Autodesk Inventor part; units mm, degrees
ref_plane "YZ Plane" through (0, 0, 0) normal (1, 0, 0) x (0, 1, 0)
ref_plane "XY Plane" through (0, 0, 0) normal (0, 0, 1) x (1, 0, 0)
sketch "Sketch1" plane through (0, 0, 0) normal (1, 0, 0) x (0, 1, 0)
  line L0 (0, -54.8873) -> (0, 55.2482)
  line L1 (0, 55.8624) -> (24.75, 55.8624)
  line L2 (24.75, 55.8624) -> (24.75, -93.6376)
  line L3 (24.75, -93.6376) -> (7.5, -93.6376)
  line L4 (7.5, -93.6376) -> (7.5, -96.6376)
  line L5 (7.5, -96.6376) -> (10, -98.6376)
  line L6 (10, -98.6376) -> (10, -99.6376)
  line L7 (10, -99.6376) -> (0, -99.6376)
  line L8 (0, -99.6376) -> (0, 55.8624)
  point P0 (0, 0)
  dimension "d0" = 155.5
  dimension "d1" = 24.75
  dimension "d2" = 7.5
  dimension "d3" = 10
  dimension "d4" = 6
  dimension "d5" = 1
  dimension "d6" = 2
revolve "Revolution1" add sketch "Sketch1" angle 360 about axis through (0, 0, -54.8873) along (0, 0, 1)
hole "Hole1" at (0, 0, -99.6376) direction (0, 0, 1) diameter 6 depth 53.5
properties part number "solenoid_body"
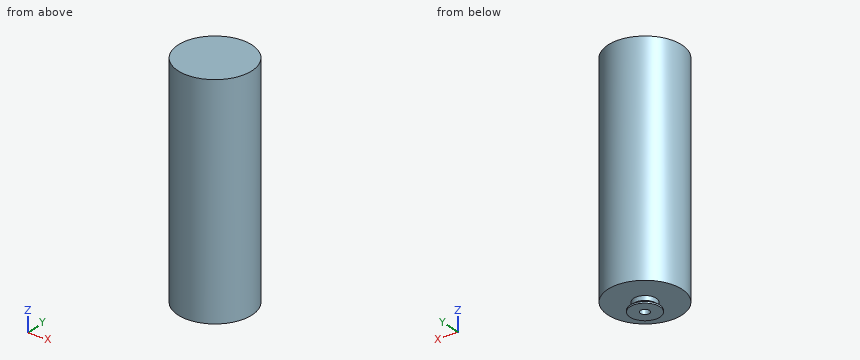
Design review of the part built by this model. Coordinates are the model's own, in mm. Give positions to 0.01 mm unless a question says otherwise; leave off trailing zeros. Order: outer loops, then holes, each group sorted by start corner. A loop starts at its lowest first (then second) coordinate and runs counter-clockwise, first axis right, second up. Notation, with made-up numbers: (8.5, 4.25) - (25.5, 4.25) arc R35 cw to (25.5, 42.25) - close; hole circle Ø1 at (34.5, 33). An arc over 180 degrees is marked (long way). Use a Markdown table: item, result. Add a question column.
(1) Clearance check with flat-ended pins moving along their axes: P1, Ø6, axis at y = 1.5, z = 0, coming from the -X side; P2, Ø1, axis at x = 14.5, z = -44, coming from the -Y side; P3, Ø3, axis at y = 12.5, z = -81, coming from the +X side; P4, Ø15, axis at x = 11, y = 5.5, coming from the -Z side. State where each tip first meets the part, or that it passes through.
(2) Wall thickness on probe 1 along X at (y, z) = (0, -71); probe 2 along Z at (x, y) = (12, -16.5): over which ranges is each line inside the solid? List them lowest first. Write a range as [from, to].
(3) Add section D-D on z = -12.5. Give the boundary of the cut face in (x, y).
(4) Add section A-A on y = 0. Give the boundary of the cut face in (x, z), then the cut area to 3 significant figures.
(5) Add section C-C on z = -49.5. Give the boundary of the cut face in (x, y).
Report:
| question | item | result |
|---|---|---|
| 1 | P1 | stops at x = -24.75 |
| 1 | P2 | stops at y = -20.41 |
| 1 | P3 | stops at x = 22.17 |
| 1 | P4 | stops at z = -99.64 |
| 2 | probe 1 | x = [-24.75, -3], [3, 24.75] |
| 2 | probe 2 | z = [-93.64, 55.86] |
| 3 | outline | circle Ø49.5 at (0, 0) |
| 4 | outline | (-24.75, -93.64) - (-7.5, -93.64) - (-7.5, -96.64) - (-10, -98.64) - (-10, -99.64) - (-3, -99.64) - (-3, -46.14) - (3, -46.14) - (3, -99.64) - (10, -99.64) - (10, -98.64) - (7.5, -96.64) - (7.5, -93.64) - (24.75, -93.64) - (24.75, 55.86) - (-24.75, 55.86) - close |
| 4 | area | 7,180 mm² |
| 5 | outline | circle Ø49.5 at (0, 0); hole circle Ø6 at (0, 0) |
